from build123d import *

# Parameters (mm, degrees)
F0_W     = 23.5
F0_H     = 44
F1_DEPTH = 8
F2_W     = 10
F2_H     = 12
F3_DEPTH = 8
F4_W     = 7.5
F4_H     = 6
F5_DEPTH = 1
F7_DEPTH = 7


with BuildPart() as f1:
    # F0 (on Front) → F1 (new body)
    with BuildSketch(Plane.XZ):
        Rectangle(F0_W, F0_H)
    extrude(amount=F1_DEPTH)

    # F2 (on face) → F3 (cut, through all)
    with BuildSketch(Plane.XZ.offset(8)):
        with Locations((-6.75, 16)):
            Rectangle(F2_W, F2_H)
        with Locations((6.75, -16)):
            Rectangle(F2_W, F2_H)
        Polygon((11.75, 16), (11.75, 22), (5.75, 22), (5.75, 16), (11.75, 10), align=None)
        Polygon((-11.75, -16), (-11.75, -22), (-5.75, -22), (-5.75, -16), (-11.75, -10), align=None)
    extrude(amount=-F3_DEPTH, mode=Mode.SUBTRACT)

    # F4 (on face) → F5 (cut)
    with BuildSketch(Plane.XZ.offset(8)):
        Polygon((-0.25, 4.21563), (11.75, 6.961239), (11.75, 8.5), (-1.305453, 5.512903), (-3.873864, -0.090707), (-11.75, -3.5), (-11.75, -5.134498), (-2.75, -1.238726), align=None)
        Polygon((0.86777, 2.841763), (-1.55978, -2.454526), (-11.75, -6.865502), (-11.75, -8.5), (-0.435916, -3.602545), (1.923223, 1.54449), (11.75, 3.792863), (11.75, 5.331624), align=None)
        with Locations((2, 19)):
            Rectangle(F4_W, F4_H)
        with Locations((-2, -19)):
            Rectangle(F4_W, F4_H)
    extrude(amount=-F5_DEPTH, mode=Mode.SUBTRACT)

    # F6 (on face) → F7 (cut, through all)
    with BuildSketch(Plane.XZ.offset(7)):
        Polygon((11.75, 6.961239), (11.75, 8.5), (10.75, 8.271199), (10.75, 6.732438), align=None)
        Polygon((11.75, 3.792863), (11.75, 5.331624), (10.75, 5.102824), (10.75, 3.564062), align=None)
        Polygon((-11.75, -3.5), (-11.75, -5.134498), (-10.75, -4.701635), (-10.75, -3.067136), align=None)
        Polygon((-11.75, -6.865502), (-11.75, -8.5), (-10.75, -8.067136), (-10.75, -6.432638), align=None)
    extrude(amount=-F7_DEPTH, mode=Mode.SUBTRACT)


solid = f1.part
Check sheet for the modelled part. Datum: model origin and axes. Units: mm. A direction names the side the tool comes from. Round coordinates to 2 decimals unless told otherwise and drop trailing zeros. Loops run counter-clockwise (first coordinate to the right, second up) from the corner with the lowest first, then second, coordinate; pieces in that order, holes last.
1. Gauge pin test, flat ends, axial feed: pin 1 Ø0.8 at (x, y) = (3.5, -7.5) entering from +Z; pin 2 Ø2 at (y, z) = (-2.5, -4.5) entering from -X; pin 3 Ø2.5 at (x, y) = (-5, -2.5) entering from +Z; pin 4 Ø1 at (x, y) = (8, -4) entering from -Z. Record the tip position at first contact, or that the pin passes through.
2. Scan lines: probe 1 along X at (y, z) = (-5, 18); probe 2 along Z at (x, y) = (-10, -4.5); probe 3 along Z at (x, y) = (2.25, -0.25). Record each from-to range of solid material in increasing order.
3. Sectioned sample at C-C on x = -9.25. Record the boundary of the cut face in (y, z), and give its area (3 significant figures).
4. Set-up check for faces 4 (the flat face through (-1.517, -7.507, 1.45)), 5 (the flat face through (-2, -7, -19)), 6 (the flat face through (-11.257, -3.549, -4.921)): record each of +Z, -Z, +X, -X, +Y, -Y from which the full face is reachable in a straight line by a thin tool's end or side.
5. Sectioned sample at A-A on y = -1.75. Record the boundary of the cut face in (x, z).
6. Sectioned sample at B-B on x = 3.5. Record the boundary of the cut face in (y, z).
7. Mould release check, pull along X, two halves, no side actions. Record for faces 1 (the flat face through (-1, -7, 3)), 2 (the flat face through (7, -4, -10)), 3 (the flat face through (1.75, -4, -16)): released by +X, released by -X, zero draft, split by the parting line, or undercut.
8. Sectioned sample at D-D on x = -2.25. Record the boundary of the cut face in (y, z).
Recorded:
1. pin 1: stops at z = 16
1. pin 2: stops at x = -11.75
1. pin 3: stops at z = 10
1. pin 4: stops at z = -10
2. probe 1: x = -1.75 to 5.75
2. probe 2: z = -11.75 to 10
2. probe 3: z = -10 to 22
3. outline: (-8, -12.5) - (0, -12.5) - (0, 10) - (-8, 10) - (-8, -2.42) - (-7, -2.42) - (-7, -4.05) - (-8, -4.05) - (-8, -5.78) - (-7, -5.78) - (-7, -7.42) - (-8, -7.42) - close
3. area: 177 mm2
4. face 4: -Y
4. face 5: -Z, +X, -X, -Y
4. face 6: -X, +Y, -Y
5. outline: (-11.75, -10) - (-5.75, -16) - (-5.75, -22) - (1.75, -22) - (1.75, -10) - (11.75, -10) - (11.75, 3.79) - (10.75, 3.56) - (10.75, 5.1) - (11.75, 5.33) - (11.75, 6.96) - (10.75, 6.73) - (10.75, 8.27) - (11.75, 8.5) - (11.75, 10) - (5.75, 16) - (5.75, 22) - (-1.75, 22) - (-1.75, 10) - (-11.75, 10) - (-11.75, -3.5) - (-10.75, -3.07) - (-10.75, -4.7) - (-11.75, -5.13) - (-11.75, -6.87) - (-10.75, -6.43) - (-10.75, -8.07) - (-11.75, -8.5) - close
6. outline: (-8, -10) - (0, -10) - (0, 22) - (-7, 22) - (-7, 16) - (-8, 16) - (-8, 6.61) - (-7, 6.61) - (-7, 5.07) - (-8, 5.07) - (-8, 3.44) - (-7, 3.44) - (-7, 1.91) - (-8, 1.91) - close
7. face 1: undercut
7. face 2: zero draft
7. face 3: released by +X
8. outline: (-8, -16) - (-7, -16) - (-7, -22) - (0, -22) - (0, 10) - (-8, 10) - (-8, 3.45) - (-7, 3.45) - (-7, -0.15) - (-8, -0.15) - (-8, -2.75) - (-7, -2.75) - (-7, -4.39) - (-8, -4.39) - close
